Work out the finished part from the listing and answer in its coordinate system (mm). Coordinates: 2 decimals unless noted, no trailing zeros. Loops run counter-clockwise (first coordinate to the right, second up) from the corner with the lowest first, then second, coordinate; pieces in that order, holes last. Notation, with made-up numbers: (9.5, -38.5) - (15.5, -38.5) arc R18 ccw to (15.5, -5.5) - close; hole circle Ø2 at (6.25, -28). An arc over 180 degrees is marked (long way). Write each question's results on one line, items separated by ' | '. Start each with the question number.
Item 1: Consider probe 1 along Y at (x, z) = (27, 12.25); probe 2 along Y at (x, z) = (43, 12.9). Determine where each line is inside the solid, lowest interval first. Write a range as [from, to].
Item 2: Section B-B, the plane z = 9 is taken. Write down the section's boundary in (x, y), plus the area to 3 significant figures.
Item 3: Section A-A, the plane x = 35.5 is taken. Write down the section's boundary in (y, z).
from build123d import *

# Parameters (mm, degrees)
BOX_W       = 43
BOX_H       = 34
BOX_DEPTH   = 6
FILLET002_R = 2
FILLET003_R = 2


with BuildPart() as part:
    # Box → Box (new body)
    with BuildSketch(Plane.XY):
        with Locations((21.5, 17)):
            Rectangle(BOX_W, BOX_H)
    extrude(amount=BOX_DEPTH)

    # Fillet002
    fillet002_edges = [part.edges().sort_by_distance(p)[0] for p in [
        (21.5, 0, 6),
        (21.5, 0, 0),
    ]]
    fillet(fillet002_edges, radius=FILLET002_R)

    # Fillet003
    fillet003_edges = [part.edges().sort_by_distance(p)[0] for p in [
        (21.5, 34, 0),
        (21.5, 34, 6),
    ]]
    fillet(fillet003_edges, radius=FILLET003_R)


with BuildPart() as part_1:
    # Body011 placement: moved
    add(part.part.moved(Location((4, 2.5, 8))))


solid = part_1.part
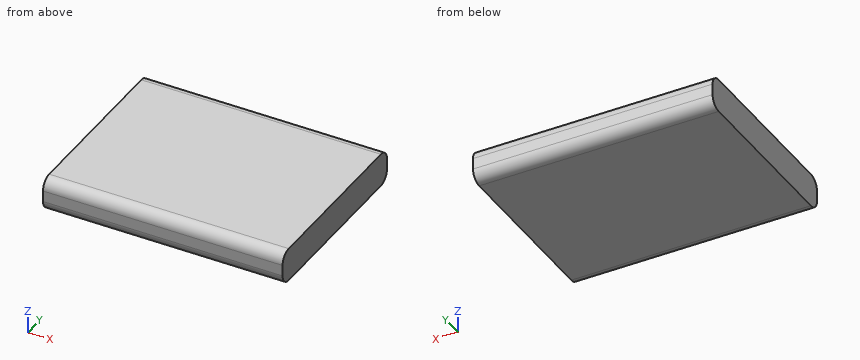
Answer key:
1) probe 1: y = [2.52, 36.48] | probe 2: y = [2.71, 36.29]
2) outline: (4, 2.77) - (47, 2.77) - (47, 36.23) - (4, 36.23) - close | area: 1,440 mm^2
3) outline: (2.5, 10) arc R2 ccw to (4.5, 8) - (34.5, 8) arc R2 ccw to (36.5, 10) - (36.5, 12) arc R2 ccw to (34.5, 14) - (4.5, 14) arc R2 ccw to (2.5, 12) - close
